Geometry: see drawing. Coordinates: mm, zero at the bounding-box minimum. A direction names the side the tool comes from. Coordinates: 2 decimals unless noted, no trailing zeros. Order: outer loops, then holes, each group sorted by start corner. A loop starts at its lowest first (then second) coordinate and runs counter-clockwise, first axis right, second up. Notation, with made-up numbers: (23, 21.25) -> (72, 21.25) arc R16 ccw to (72, 35.25) -> close; hole circle Ø1 at (34, 10). An arc over 180 degrees is marked (long way). Write each question's results on one line, items separated by ' | '.
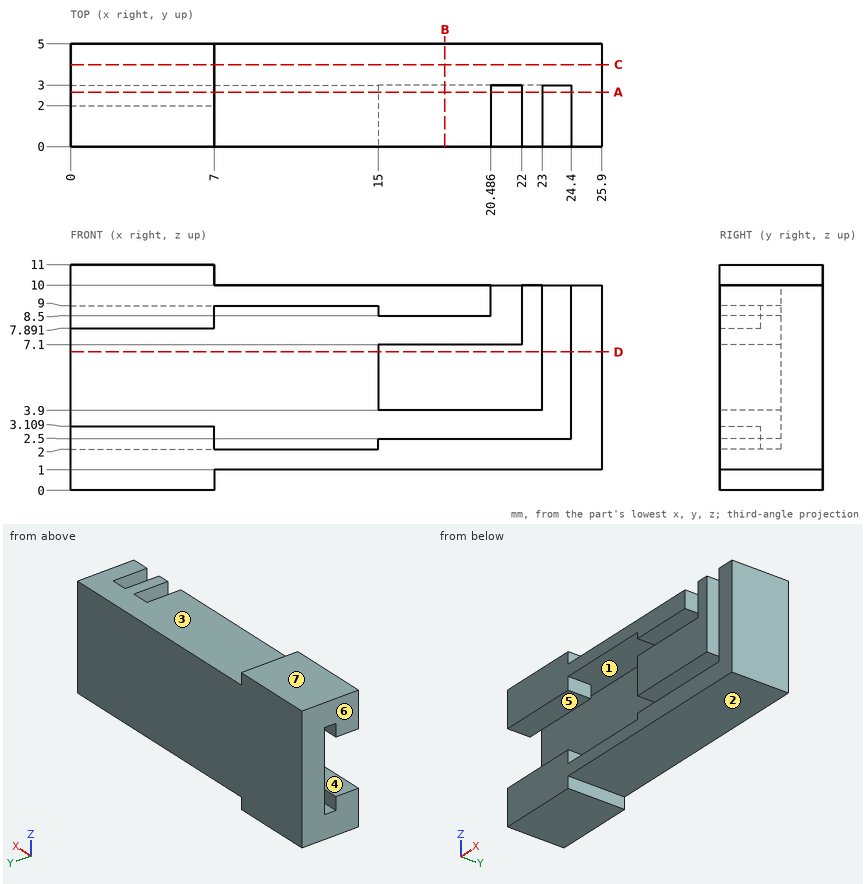
(1) Pin query (flat end, axial travel): P1, Ø1.5, axis at x = 9.5, y = 2, coming from the +Z side. Return the tip coordinate at first contact, or that it passes through.
Return value:
P1: z = 10
(2) Cut plane C-C, the plane y = 4. Return loops of the section in (x, z).
Return value:
outline: (0, 0) -> (7, 0) -> (7, 1) -> (25.9, 1) -> (25.9, 10) -> (7, 10) -> (7, 11) -> (0, 11) -> close
(3) Line query: line 1 along X through (y, z) = (2.6, 9.75); line 2 along Z through (x, y) = (19.5, 2.45); line 3 along Z through (x, y) = (2, 1.8). Output: solid intervals per line, ascending. Write a range as from..to.
Return value:
line 1: 0..20.49, 22..23, 24.4..25.9 | line 2: 1..2.5, 3.9..7.1, 8.5..10 | line 3: 0..3.11, 7.89..11
(4) Cut plane B-B, the plane x = 18.25. Return loops of the section in (y, z), plus the area to 3 significant figures.
Return value:
outline: (0, 1) -> (5, 1) -> (5, 10) -> (0, 10) -> (0, 8.5) -> (3, 8.5) -> (3, 7.1) -> (0, 7.1) -> (0, 3.9) -> (3, 3.9) -> (3, 2.5) -> (0, 2.5) -> close | area: 36.6 mm2
(5) Cut plane D-D, the plane z = 6.75. Return loops of the section in (x, y).
Return value:
outline: (0, 3) -> (15, 3) -> (15, 0) -> (23, 0) -> (23, 3) -> (24.4, 3) -> (24.4, 0) -> (25.9, 0) -> (25.9, 5) -> (0, 5) -> close
(6) Cut plane A-A, the plane y = 2.65. Return loops of the section in (x, z), plus the area to 3 significant figures.
Return value:
outline: (0, 0) -> (7, 0) -> (7, 1) -> (25.9, 1) -> (25.9, 10) -> (24.4, 10) -> (24.4, 2.5) -> (15, 2.5) -> (15, 2) -> (0, 2) -> close; (0, 9) -> (15, 9) -> (15, 8.5) -> (20.49, 8.5) -> (20.49, 10) -> (7, 10) -> (7, 11) -> (0, 11) -> close; (15, 3.9) -> (23, 3.9) -> (23, 10) -> (22, 10) -> (22, 7.1) -> (15, 7.1) -> close | area: 108 mm2
(7) Mould query, pull axis Z, two halves, no side actions, for the marked faces 5, 6 and 7. Classes: +Z half, -Z half, draft (parallel to the pull), parting line (faces both ways), or undercut.
Return value:
face 5: undercut | face 6: draft | face 7: +Z half
(8) Reachability of the marked faces 1, 2, 3 and 4 from +Z, -Z, +X, -X, +Y, -Y: full face, straight path, thin tool, end or side. Return the list, or none.
Return value:
face 1: none | face 2: -Z, +X, +Y, -Y | face 3: +Z, +X, +Y, -Y | face 4: -X, -Y
